Could you check a few things on this model? Use its own coordinates, in mm. Face numbers are marked on the shaded views. A direction names the side the tool comes from. Coordinates: 2 decimals unless noted, no trailing zeros. Order: outer loops, then holes, each group sorted by start corner. A loop starts at its lowest first (then second) coordinate and runs counter-clockwise, first axis right, second up. Notation, with made-up numbers: M 36.25,45 L 53.25,45 A13 cw 53.25,53 Z; hole C 74,29.25 d1. An arc over 180 degrees is marked long. Write item = value, one per line. Start each with the question number.
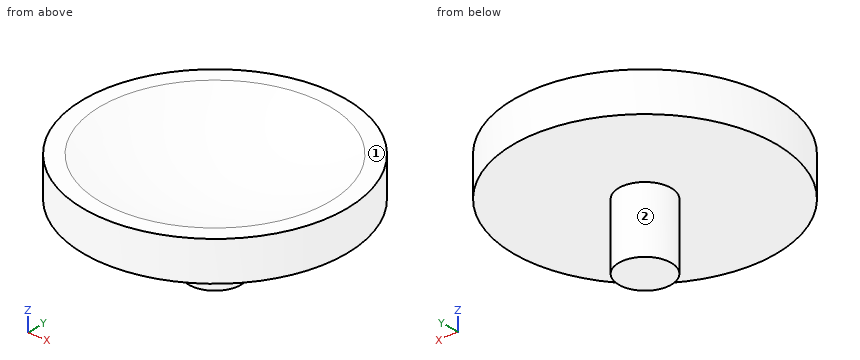
from build123d import *

# Parameters (mm, degrees)
F0_R     = 10
F1_DEPTH = 3
F4_R     = 2
F5_DEPTH = 5


with BuildPart() as f1:
    # F0 (on Top) → F1 (new body)
    with BuildSketch(Plane.XY):
        Circle(F0_R)
    extrude(amount=F1_DEPTH)

    # F2 (on Front) → F3 (revolve, cut)
    with BuildSketch(Plane.XZ):
        with BuildLine():
            Line((0, 1), (0, 41))
            ThreePointArc((0, 41), (-20, 21), (0, 1))
        make_face()
    revolve(axis=Axis((0, 0, 27.434054), (0, 0, -1)), mode=Mode.SUBTRACT)

    # F4 (on face) → F5 (join)
    with BuildSketch(Plane(origin=(0, 0, 0), x_dir=(1, 0, 0), z_dir=(0, 0, -1))):
        Circle(F4_R)
    extrude(amount=F5_DEPTH)


solid = f1.part
(1) Imagine slicing it at D-D on z = 2. List the corners of the cut face in (x, y) for me (3 decimals).
(2) Imagine slicing it at C-C on z = -1.25. List the corners of the cut face in (x, y) for me, plus the area to 3 significant figures.
(3) Imagine slicing it at A-A on y = 0. List the corners of the cut face in (x, z) for me, plus the area to 3 significant figures.
(4) Will these pins go through, and if not, where does the flat tip stop? P1, Ø4, axis at x = 7, z = 1.5, coming from the -Y side; P2, Ø3, axis at y = 2, z = -3, coming from the -X side; P3, Ø1.5, axis at x = 0.5, y = 4.5, coming from the -Z side.
(5) For the marked faces 1 and 2, which set-ups out of +Z, -Z, +X, -X, +Y, -Y let a thin tool reach every point of the face, with its end or its side?
(6) Please list where these lines run through material, in increasing order: probe 1 along Z at (x, y) = (-6.5, 7.5); probe 2 along Z at (x, y) = (-2, 2.5); probe 3 along X at (y, z) = (-1.5, -3.5). Write a range as from..to.
Response:
q1.outline = C 0,0 d20; hole C 0,0 d12.49
q2.outline = C 0,0 d4
q2.area = 12.6 mm2
q3.outline = M -10,0 L -2,0 L -2,-5 L 2,-5 L 2,0 L 10,0 L 10,3 L 8.72,3 A20 cw -8.72,3 L -10,3 Z
q3.area = 56.5 mm2
q4.P1 = -8.66
q4.P2 = -1.94
q4.P3 = 0
q5.face_1 = +Z, +X, -X, +Y, -Y
q5.face_2 = -Z
q6.probe_1 = 0..3
q6.probe_2 = 0..1.26
q6.probe_3 = -1.32..1.32
